Here's how the part is built. I have some questions about the finished solid (model axes, mm). Face numbers are marked on the shaded views. Round coordinates to 2 decimals unless told otherwise and drop trailing zeros. Loops run counter-clockwise (first coordinate to the right, second up) from the corner with the lowest first, then second, coordinate; pieces in that order, holes last. Notation, with made-up numbers: M 41,63.5 L 86,63.5 A18 cw 86,68.5 Z; hole C 48.25,-32.75 d10. An arc over 180 degrees is marked long. Write item = value, one per line. Start each with the question number.
from build123d import *

# Parameters (mm, degrees)
BOSS_EXTRU_1_DEPTH              = 1
EXTRU_MINCE1_DEPTH              = 1.5
EXTRU_MINCE1_TAPER              = -10
ENL_V_DE_MAT_EXTRU_MINCE1_DEPTH = 3.5000001
ESQUISSE4_R                     = 2.5
BOSS_EXTRU_2_DEPTH              = 3.8


with BuildPart() as part:
    # Esquisse1 → Boss.-Extru.1 (new body)
    with BuildSketch(Plane.XY):
        Polygon((-59.024791386, -44.744645862), (2.7, -44.744645862), (59.024791386, -44.744645862), (68.262395693, -28.744645862), (51.666666667, 0), (-51.666666667, 0), (-68.262395693, -28.744645862), align=None)
    extrude(amount=BOSS_EXTRU_1_DEPTH)

    # Esquisse2 → Extru.-Mince1 (add)
    with BuildSketch(Plane.XY.offset(1)):
        Polygon((-68.262395693, -28.744645862), (-59.024791386, -44.744645862), (59.024791386, -44.744645862), (68.262395693, -28.744645862), (51.666666667, 0), (-51.666666667, 0), align=None)
        Polygon((-66.183934724, -28.744645862), (-57.985560901, -42.944645862), (57.985560901, -42.944645862), (66.183934724, -28.744645862), (50.627436182, -1.8), (-50.627436182, -1.8), align=None, mode=Mode.SUBTRACT)
    extrude(amount=EXTRU_MINCE1_DEPTH, taper=EXTRU_MINCE1_TAPER)

    # Esquisse3 → Enlèv. de mat.-Extru.-Mince1 (cut, through all)
    with BuildSketch(Plane(origin=(0, 0, 0), x_dir=(-1, 0, 0), z_dir=(0, 0, -1))):
        Polygon((60.121756897, -46.644645862), (70.456326716, -28.744645862), (52.763632178, 1.9), (-52.763632178, 1.9), (-70.456326716, -28.744645862), (-60.121756897, -46.644645862), align=None)
        Polygon((59.024791386, -44.744645862), (68.262395693, -28.744645862), (51.666666667, 0), (-51.666666667, 0), (-68.262395693, -28.744645862), (-59.024791386, -44.744645862), align=None, mode=Mode.SUBTRACT)
    extrude(amount=-ENL_V_DE_MAT_EXTRU_MINCE1_DEPTH, mode=Mode.SUBTRACT)

    # Esquisse4 → Boss.-Extru.2 (add)
    with BuildSketch(Plane.XY.offset(1)):
        with Locations((25.665479371, -13.424541306)):
            Circle(ESQUISSE4_R)
    extrude(amount=BOSS_EXTRU_2_DEPTH)


solid = part.part
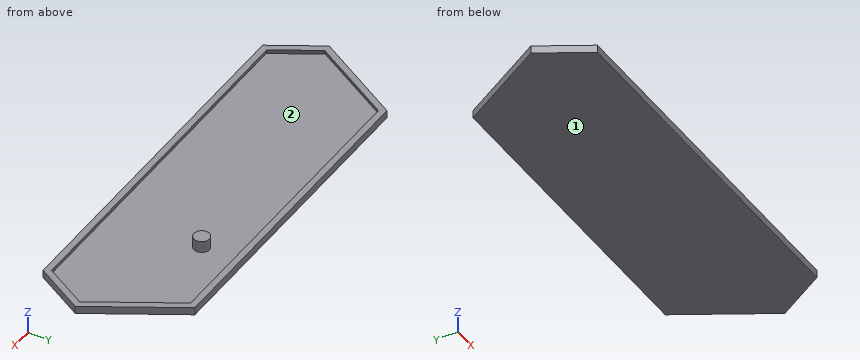
Item 1: Will this pin go through, and if not, where does the flat tip stop? pin 1 Ø8 at (x, y) = (-50.5, -16.5) entering from +Z.
Item 2: Please list where these lines run through material, in increasing order: line 1 (X direction, y = -12, z = 1.2); line 2 (Z direction, x = 43.5, y = -31); line 3 (X direction, y = -13, z = 1.55). Write a range as [from, to].
Item 3: I want a section at A-A, the plane z = 3.6. List the corners of the cut face in (x, y) for me.
Item 4: We'd pull the mould along X, two halves only. Please class the marked faces 1 and 2: released by +X, released by -X, zero draft, split by the parting line, or undercut.
Worked out:
q1.pin_1 = 1
q2.line_1 = [-58.59, -56.48], [23.61, 27.72], [56.48, 58.59]
q2.line_2 = [0, 1]
q2.line_3 = [-59.17, -56.98], [23.2, 28.13], [56.98, 59.17]
q3.outline = C 25.67,-13.42 d5
q4.face_1 = zero draft
q4.face_2 = undercut
